Autodesk Inventor part; units mm, degrees
ref_plane "YZ Plane" through (0, 0, 0) normal (1, 0, 0) x (0, 1, 0)
ref_plane "XZ Plane" through (0, 0, 0) normal (0, 1, 0) x (-1, 0, 0)
ref_plane "XY Plane" through (0, 0, 0) normal (0, 0, 1) x (1, 0, 0)
sketch "Sketch1" plane through (0, 0, 0) normal (0, 1, 0) x (-1, 0, 0)
  line L0 (-254, 304.8) -> (254, 304.8)
  line L1 (254, 304.8) -> (254, -304.8)
  line L2 (254, -304.8) -> (-254, -304.8)
  line L3 (-254, -304.8) -> (-254, 304.8)
  line L4 (-254, 304.8) -> (254, -304.8) construction
  line L5 (254, 304.8) -> (-254, -304.8) construction
  point P0 (0, 0)
  dimension "d0" = 609.6
  dimension "d1" = 508
extrude "Extrusion1" add sketch "Sketch1" along normal blind 50.8
chamfer "Chamfer1" distance 50.8 angle 45 4 edges at (254, 50.8, 0) (0, 50.8, -304.8) (-254, 50.8, 0) (0, 50.8, 304.8)
properties part number "hologram display base (for assembly)"
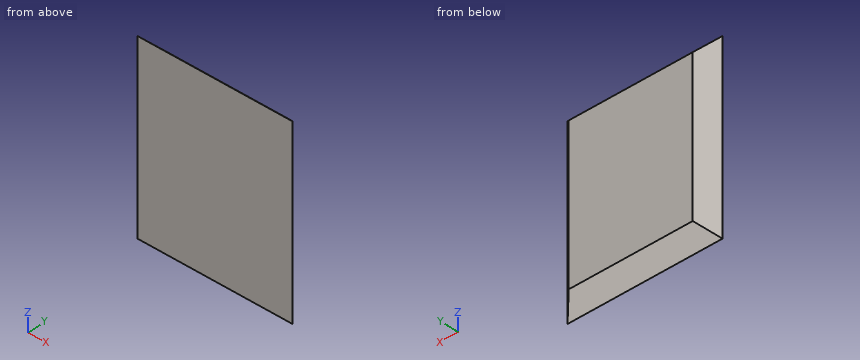
Input: part model. Units: mm. Frame: model coordinates. Give positions to 0.01 mm unless a question says otherwise; leave off trailing zeros. Loops run counter-clockwise (first coordinate to the right, second up) from the corner with the lowest first, then second, coordinate; pieces in that order, holes last. Notation, with made-up numbers: M 45.25,-11.75 L 91.25,-11.75 A9 ccw 91.25,0.25 Z; hole C 42,11 d11. An arc over 180 degrees is marked long. Use CSV: the item, a comma, the result in double quotes.
(1) Pin query (flat end, axial travel): P1, Ø10, axis at y = 40, z = -131, coming from the +X side; P2, Ø2, axis at x = 146, y = 6, coming from the -Z side; P3, Ø8, axis at y = 43, z = -199, coming from the +X side; P4, Ø12, axis at x = 179, z = -221.5, coming from the -Y side. Return the tip coordinate at first contact, or that it passes through.
Outcome:
P1,"stops at x = 219"
P2,"stops at z = -299.8"
P3,"stops at x = 215"
P4,"stops at y = 0"
(2) Section C-C, the plane y = 32.5. Return loops of the section in (x, z), plus the area to 3 significant figures.
Outcome:
outline,"M -221.5,-272.3 L 221.5,-272.3 L 221.5,272.3 L -221.5,272.3 Z"
area,"241,000 mm²"
(3) Material intervals for L1, parallel to X at y = 5, z = -2.5; L2, parallel to X at y = 32, z = 18; L3, parallel to Z at x = 106.5, y = 11, sorted ascending. Write a range as [from, to].
Outcome:
L1,"x = [-249, 249]"
L2,"x = [-222, 222]"
L3,"z = [-293.8, 293.8]"
